Geometry check sheet. Reference: drawing and pictorial views, mm from the part's lowest x, y, z. Round coordinates to 2 decimals unless told otherwise and drop trailing zeros. Order: outer loops, then holes, each group sorted by start corner. A loop starts at its lowest first (then second) coordinate and runs counter-clockwise, first axis right, second up.
(1) Sectioned sample at C-C, the plane x = 2.5. Enter the section's corners in (y, z).
(2) Sectioned sample at D-D, the plane z = 7. Enter the section's corners in (x, y), and give its area (3 significant figures).
(3) Mould release check, pull along X, two halves, no side actions. Record for the marked faces 1, 2, 3 and 4: released by +X, released by -X, zero draft, split by the parting line, or undercut.
(4) Sectioned sample at A-A, the plane y = 3. Enter the section's corners in (x, z), and give its area (3 significant figures).
(5) Sectioned sample at B-B, the plane y = 4.5. Enter the section's corners in (x, z), and give its area (3 significant figures).
(6) Depth check by flat-ended pin: pin 1 (1.6 mm diameter, centred on x = 14.5, z = 7, fed in from +Y). Enter the tip coordinate at first touch or a pass-through.
(7) Thickness scan on probe 1 along X at (y, z) = (5.65, 15); probe 2 along Z at (x, y) = (14.5, 4.4); probe 3 along X at (y, z) = (3.25, 5). Record the ranges inside material, lowest first.
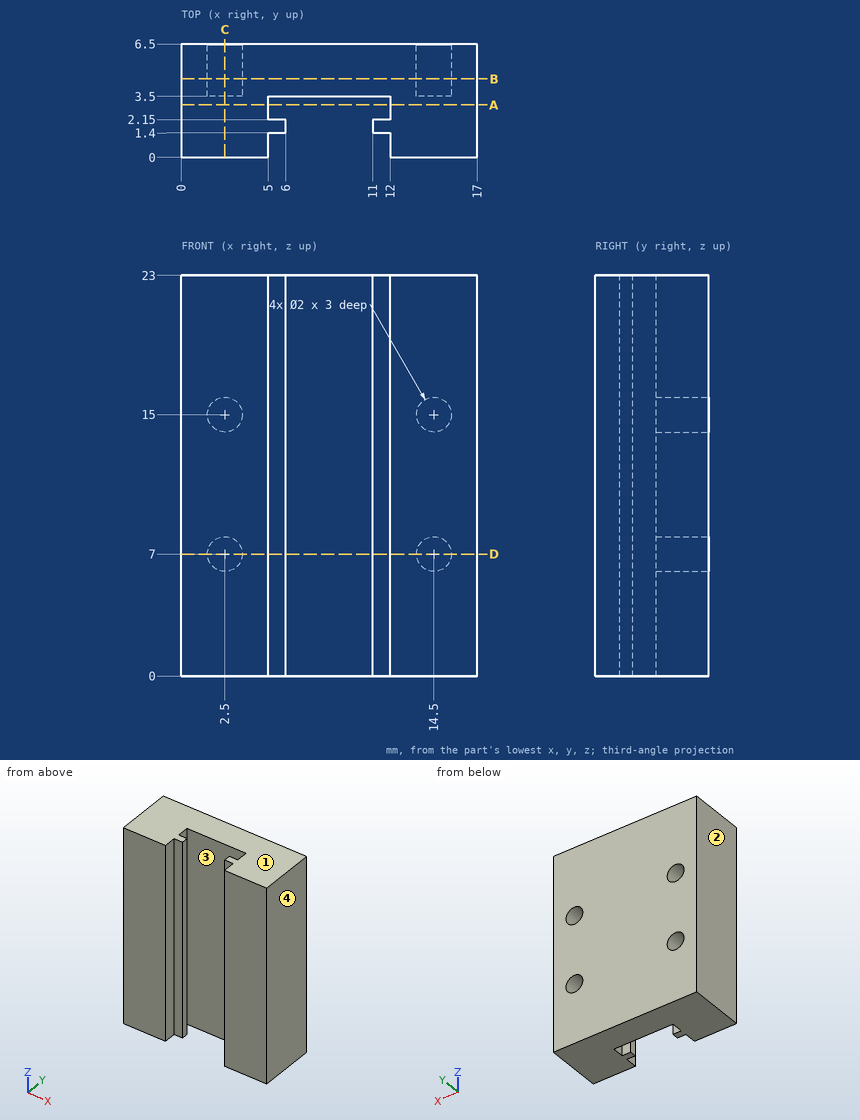
Derived:
1. outline: (0, 0) - (6.5, 0) - (6.5, 6) - (3.5, 6) - (3.5, 8) - (6.5, 8) - (6.5, 14) - (3.5, 14) - (3.5, 16) - (6.5, 16) - (6.5, 23) - (0, 23) - close
2. outline: (0, 0) - (5, 0) - (5, 1.4) - (6, 1.4) - (6, 2.15) - (5, 2.15) - (5, 3.5) - (12, 3.5) - (12, 2.15) - (11, 2.15) - (11, 1.4) - (12, 1.4) - (12, 0) - (17, 0) - (17, 6.5) - (15.5, 6.5) - (15.5, 3.5) - (13.5, 3.5) - (13.5, 6.5) - (3.5, 6.5) - (3.5, 3.5) - (1.5, 3.5) - (1.5, 6.5) - (0, 6.5) - close
2. area: 75.5 mm2
3. face 1: zero draft
3. face 2: released by -X
3. face 3: undercut
3. face 4: released by +X
4. outline: (0, 0) - (5, 0) - (5, 23) - (0, 23) - close; (12, 0) - (17, 0) - (17, 23) - (12, 23) - close
4. area: 230 mm2
5. outline: (0, 0) - (17, 0) - (17, 23) - (0, 23) - close; hole circle Ø2 at (2.5, 7); hole circle Ø2 at (2.5, 15); hole circle Ø2 at (14.5, 7); hole circle Ø2 at (14.5, 15)
5. area: 378 mm2
6. pin 1: stops at y = 3.5
7. probe 1: x = 0 to 1.5, 3.5 to 13.5, 15.5 to 17
7. probe 2: z = 0 to 6, 8 to 14, 16 to 23
7. probe 3: x = 0 to 5, 12 to 17
